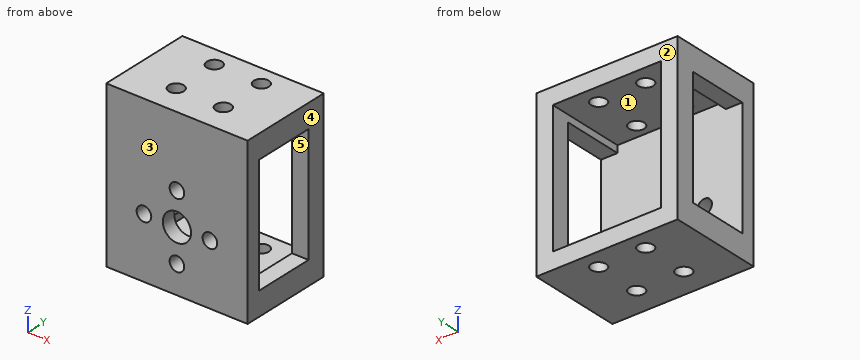
from build123d import *

# Parameters (mm, degrees)
SKETCH_1_W          = 23
SKETCH_1_H          = 35
EXTRUDE_2_DEPTH     = 3
EXTRUDE_3_DEPTH     = 18
EXTRUDE_3_2_DEPTH   = 18
EXTRUDE_4_DEPTH     = 20
CUT_EXTRUDE_5_DEPTH = 31
SKETCH_9_R          = 1.55
SKETCH_9_R_2        = 3
CUT_EXTRUDE_6_DEPTH = 21
SKETCH_10_R         = 1.6
CUT_EXTRUDE_7_DEPTH = 36


with BuildPart() as part:
    # Sketch 1 → Extrude 2 (new body)
    with BuildSketch(Plane(origin=(0, 0, 0), x_dir=(1, 0, 0), z_dir=(0, 1, 0))):
        Rectangle(SKETCH_1_W, SKETCH_1_H)
    extrude(amount=EXTRUDE_2_DEPTH)



with BuildPart() as body_2:
    # Sketch 1_4 → Extrude 3 (new body)
    with BuildSketch(Plane(origin=(0, 0, 0), x_dir=(1, 0, 0), z_dir=(0, 1, 0))):
        Polygon((11.5, -17.5), (11.5, -14), (0, -14), (-8.5, -14), (-11.5, -14), (-11.5, -17.5), align=None)
    extrude(amount=EXTRUDE_3_DEPTH)


with BuildPart() as body_3:
    # Sketch 1_4 → Extrude 3 2 (new body)
    with BuildSketch(Plane(origin=(0, 0, 0), x_dir=(1, 0, 0), z_dir=(0, 1, 0))):
        Polygon((-11.5, 14), (0, 14), (11.5, 14), (11.5, 17.5), (-11.5, 17.5), align=None)
    extrude(amount=EXTRUDE_3_2_DEPTH)


with BuildPart() as part_1:
    add(part.part)

    add(body_2.part)  # Extrude 4 merges body 2

    add(body_3.part)  # Extrude 4 merges body 3
    # Sketch 1_5 → Extrude 4 (add)
    with BuildSketch(Plane(origin=(0, 0, 0), x_dir=(1, 0, 0), z_dir=(0, 1, 0))):
        Polygon((-11.5, 0), (-11.5, 14), (-11.5, 17.5), (-15, 17.5), (-15, -17.5), (-11.5, -17.5), (-11.5, -14), align=None)
        Polygon((11.5, 17.5), (11.5, 14), (11.5, 0), (11.5, -14), (11.5, -17.5), (15, -17.5), (15, 17.5), align=None)
        Polygon((11.5, -17.5), (11.5, -14), (0, -14), (-8.5, -14), (-11.5, -14), (-11.5, -17.5), align=None)
        Polygon((-11.5, 14), (0, 14), (11.5, 14), (11.5, 17.5), (-11.5, 17.5), align=None)
    extrude(amount=EXTRUDE_4_DEPTH)

    # Sketch 8 → Cut-Extrude 5 (cut, through all)
    with BuildSketch(Plane.ZY.offset(15)):
        Polygon((12.5, 3), (12.5, 10), (12.5, 16), (-12.5, 16), (-12.5, 3), (0, 3), align=None)
    extrude(amount=-CUT_EXTRUDE_5_DEPTH, mode=Mode.SUBTRACT)

    # Sketch 9 → Cut-Extrude 6 (cut, through all)
    with BuildSketch(Plane.XZ):
        with Locations((0, -11.5)):
            Circle(SKETCH_9_R)
        with Locations((0, 2.5)):
            Circle(SKETCH_9_R)
        with Locations((7, -4.5)):
            Circle(SKETCH_9_R)
        with Locations((-7, -4.5)):
            Circle(SKETCH_9_R)
        with Locations((0, -4.5)):
            Circle(SKETCH_9_R_2)
    extrude(amount=-CUT_EXTRUDE_6_DEPTH, mode=Mode.SUBTRACT)

    # Sketch 10 → Cut-Extrude 7 (cut, through all)
    with BuildSketch(Plane(origin=(0, 0, -17.5), x_dir=(-1, 0, 0), z_dir=(0, 0, -1))):
        with Locations((5, 6)):
            Circle(SKETCH_10_R)
        with Locations((-5, 6)):
            Circle(SKETCH_10_R)
        with Locations((-5, 16)):
            Circle(SKETCH_10_R)
        with Locations((5, 16)):
            Circle(SKETCH_10_R)
    extrude(amount=-CUT_EXTRUDE_7_DEPTH, mode=Mode.SUBTRACT)


solid = part_1.part
Geometry: final body of the model. Coordinates: model frame, mm. Face numbers are marked on the shaded views. A direction names the side the tool comes from. Give positions to 0.01 mm unless a question says otherwise; leave off trailing zeros. Write each loop counter-clockwise with the first axis right and the second up, starting at its lowest first coordinate (ties: lowest second). Pieces come first, ordered by that corner, then holes. Notation, with made-up numbers: (88.5, 82.25) - (146.5, 82.25) arc R22 cw to (146.5, 106.25) - close; hole circle Ø9 at (-21.5, 89). An arc over 180 degrees is marked (long way). Return JSON: item names as keys, results as strings. Group by question number.
1) Mould query, pull axis Y, two halves, no side actions, for the marked faces 3, 4 and 5. Classes: released by +Y, released by -Y, zero draft, split by the parting line, or undercut.
2) Section C-C on x = -5. Return the cut outline in (y, z).
3) Set-up query: the marked faces 1 and 2. Return all of +Z, -Z, +X, -X, +Y, -Y with unobstructed straight access to the full face (end or side cutting, diameter ignored); none if empty.
4) First-contact query: P1, Ø5, axis at x = -7, z = 10, coming from the +Y side; P2, Ø3, axis at x = -7, z = -4.5, coming from the -Y side. Flat tips, straight axial feed; report the tip coordinate or a pass-through.
5) Section A-A on x = 0. Return the cut outline in (y, z), plus the area to 3 significant figures.
6) Section D-D on y = 2.5. Return the cut outline in (x, z), plus the area to 3 significant figures.
7) Section B-B on z = -4.5. Return the cut outline in (x, y), plus the area to 3 significant figures.
8) Line query: line 1 (Y direction, x = -5, z = 15.5); line 2 (Y direction, x = 11.75, z = -8); line 3 (Z direction, x = 0.75, y = 12). Output: solid intervals per line, ascending.
Filled in:
{
 "1": {"face 3": "released by -Y", "face 4": "zero draft", "face 5": "undercut"},
 "2": {"outline": "(0, -17.5) - (4.4, -17.5) - (4.4, -14) - (3, -14) - (3, 14) - (4.4, 14) - (4.4, 17.5) - (0, 17.5) - close; (7.6, -17.5) - (14.4, -17.5) - (14.4, -14) - (7.6, -14) - close; (7.6, 14) - (14.4, 14) - (14.4, 17.5) - (7.6, 17.5) - close; (17.6, -17.5) - (20, -17.5) - (20, -14) - (17.6, -14) - close; (17.6, 14) - (20, 14) - (20, 17.5) - (17.6, 17.5) - close"},
 "3": {"face 1": "+Y", "face 2": "+Z, -Z, +X, -X, +Y"},
 "4": {"P1": "stops at y = 3", "P2": "passes through"},
 "5": {"outline": "(0, -17.5) - (20, -17.5) - (20, -14) - (3, -14) - (3, -13.05) - (0, -13.05) - close; (0, -9.95) - (3, -9.95) - (3, -7.5) - (0, -7.5) - close; (0, -1.5) - (3, -1.5) - (3, 0.95) - (0, 0.95) - close; (0, 4.05) - (3, 4.05) - (3, 14) - (20, 14) - (20, 17.5) - (0, 17.5) - close", "area": "187 mm^2"},
 "6": {"outline": "(-15, -17.5) - (15, -17.5) - (15, 17.5) - (-15, 17.5) - close; hole circle Ø3.1 at (-7, -4.5); hole circle Ø6 at (0, -4.5); hole circle Ø3.1 at (0, -11.5); hole circle Ø3.1 at (0, 2.5); hole circle Ø3.1 at (7, -4.5)", "area": "992 mm^2"},
 "7": {"outline": "(-15, 0) - (-8.55, 0) - (-8.55, 3) - (-15, 3) - close; (-15, 16) - (-11.5, 16) - (-11.5, 20) - (-15, 20) - close; (-5.45, 0) - (-3, 0) - (-3, 3) - (-5.45, 3) - close; (3, 0) - (5.45, 0) - (5.45, 3) - (3, 3) - close; (8.55, 0) - (15, 0) - (15, 3) - (8.55, 3) - close; (11.5, 16) - (15, 16) - (15, 20) - (11.5, 20) - close", "area": "81.4 mm^2"},
 "8": {"line 1": "y = 0 to 4.4, 7.6 to 14.4, 17.6 to 20", "line 2": "y = 0 to 3, 16 to 20", "line 3": "z = -17.5 to -14, 14 to 17.5"}
}
